from build123d import *

# Parameters (mm, degrees)
SKETCH1_R               = 60.625
SKETCH1_R_2             = 45
BOSS_EXTRUDE1_DEPTH     = 4
SKETCH2_R               = 49
SKETCH2_R_2             = 45
BOSS_EXTRUDE2_DEPTH     = 52
SKETCH4_W               = 13.25
SKETCH4_H               = 8
SKETCH4_W_2             = 8
SKETCH4_H_2             = 38
BOSS_EXTRUDE4_DEPTH     = 13
BOSS_EXTRUDE5_DEPTH     = 4
SKETCH7_R               = 1.3
CUT_EXTRUDE4_DEPTH      = 7.2
SKETCH9_W               = 10
SKETCH9_H               = 24
CUT_EXTRUDE7_DEPTH      = 8
CUT_EXTRUDE8_REACH      = 139.219
CUT_EXTRUDE8_END_RADIUS = 45
SKETCH11_R              = 5
CUT_EXTRUDE9_DEPTH      = 101.273532203


with BuildPart() as part:
    # Sketch1 → Boss-Extrude1 (new body)
    with BuildSketch(Plane(origin=(0, 0, 0), x_dir=(1, 0, 0), z_dir=(0, 1, 0))):
        with Locations(Location((0, 0, 0), (0, 0, 270))):
            Circle(SKETCH1_R)
        with Locations(Location((0, 0, 0), (0, 0, 270))):
            Circle(SKETCH1_R_2, mode=Mode.SUBTRACT)
    extrude(amount=BOSS_EXTRUDE1_DEPTH)

    # Sketch2 → Boss-Extrude2 (add)
    with BuildSketch(Plane(origin=(0, 4, 0), x_dir=(1, 0, 0), z_dir=(0, 1, 0))):
        with Locations(Location((0, 0, 0), (0, 0, 90))):
            Circle(SKETCH2_R)
        with Locations(Location((0, 0, 0), (0, 0, 270))):
            Circle(SKETCH2_R_2, mode=Mode.SUBTRACT)
    extrude(amount=BOSS_EXTRUDE2_DEPTH)

    # Sketch4 → Boss-Extrude4 (add, symmetric)
    with BuildSketch(Plane.XY):
        with Locations((-38.375, 34)):
            Rectangle(SKETCH4_W, SKETCH4_H)
        Polygon((-31.75, 30), (-45, 30), (-45, 16.75), align=None)
        with Locations((15.25, 19)):
            Rectangle(SKETCH4_W_2, SKETCH4_H_2)
    extrude(amount=BOSS_EXTRUDE4_DEPTH, both=True)


with BuildPart() as boss_extrude4_piece_1:
    # of the separate pieces the step leaves, piece 1, a body of its own (boss_extrude4_pieces)
    add(part.part.solids().sort_by_distance((0, 0, 60.625))[0])



with BuildPart() as boss_extrude4_piece_2:
    # of the separate pieces the step leaves, piece 2, a body of its own (boss_extrude4_pieces)
    add(part.part.solids().sort_by_distance((11.25, 38, -13))[0])


with BuildPart() as boss_extrude4_piece_1_1:
    add(boss_extrude4_piece_1.part)

    add(boss_extrude4_piece_2.part)  # Boss-Extrude5 merges Boss-Extrude4 piece 2
    # Sketch5 → Boss-Extrude5 (add)
    with BuildSketch(Plane.XZ):
        with BuildLine():
            Line((11.25, 13), (29.067400866, 34.352382842))
            ThreePointArc((29.067400866, 34.352382842), (45, 0), (29.067400866, -34.352382842))
            Line((29.067400866, -34.352382842), (11.25, -13))
            Line((11.25, -13), (11.25, 13))
        make_face()
    extrude(amount=-BOSS_EXTRUDE5_DEPTH)

    # Sketch7 → Cut-Extrude4 (cut)
    with BuildSketch(Plane(origin=(0, 38, 0), x_dir=(1, 0, 0), z_dir=(0, 1, 0))):
        with Locations(Location((-34.25, 5, 0), (0, 0, 180))):
            Circle(SKETCH7_R)
        with Locations(Location((-34.25, -5, 0), (0, 0, 180))):
            Circle(SKETCH7_R)
        with Locations(Location((13.75, 5, 0), (0, 0, 180))):
            Circle(SKETCH7_R)
        with Locations(Location((13.75, -5, 0), (0, 0, 180))):
            Circle(SKETCH7_R)
    extrude(amount=-CUT_EXTRUDE4_DEPTH, mode=Mode.SUBTRACT)

    # Sketch9 → Cut-Extrude7 (cut)
    with BuildSketch(Plane.ZY.offset(-11.25)):
        with Locations((0, 17)):
            Rectangle(SKETCH9_W, SKETCH9_H)
    extrude(amount=-CUT_EXTRUDE7_DEPTH, mode=Mode.SUBTRACT)

    # Cut-Extrude8: up to this cylinder (the profile starts outside it)
    cut_extrude8_end = Plane(origin=(0, 14, 0), z_dir=(0, -1, 0)) * Cylinder(CUT_EXTRUDE8_END_RADIUS, 369.438, mode=Mode.PRIVATE)
    # Sketch11 → Cut-Extrude8 (cut, up to the surface)
    with BuildSketch(Plane(origin=(49, 0, 0), x_dir=(0, 0, -1), z_dir=(1, 0, 0)), mode=Mode.PRIVATE) as cut_extrude8_sk1:
        with Locations((0, 14)):
            Circle(SKETCH11_R)
    cut_extrude8_tool1 = extrude(cut_extrude8_sk1.sketch, amount=-CUT_EXTRUDE8_REACH, mode=Mode.PRIVATE) - cut_extrude8_end
    add(cut_extrude8_tool1.solids().sort_by_distance((49, 14, 0))[0], mode=Mode.SUBTRACT)

    # Sketch12 → Cut-Extrude9 (cut, through all)
    with BuildSketch(Plane(origin=(0, 4, 0), x_dir=(1, 0, 0), z_dir=(0, 1, 0))):
        with BuildLine():
            Line((29.479537487, 22.359715328), (27.25, 19.687836398))
            Line((27.25, 19.687836398), (27.25, -19.687836398))
            Line((27.25, -19.687836398), (29.479537487, -22.359715328))
            ThreePointArc((29.479537487, -22.359715328), (37, 0), (29.479537487, 22.359715328))
        make_face()
        Polygon((27.25, -19.687836398), (27.25, 19.687836398), (24.25, 16.092634774), (24.25, -16.092634774), align=None)
    extrude(amount=-CUT_EXTRUDE9_DEPTH, mode=Mode.SUBTRACT)


solid = boss_extrude4_piece_1_1.part
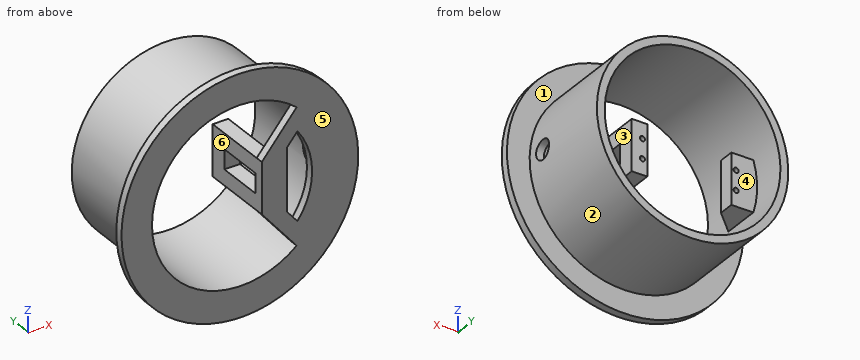
Design review of the part built by this model. Coordinates are the model's own, in mm. Face numbers are marked on the shaded views. A direction names the side the tool comes from. Give positions to 0.01 mm unless a question says otherwise; leave off trailing zeros. Loops run counter-clockwise (first coordinate to the right, second up) from the corner with the lowest first, then second, coordinate; pieces in that order, holes last. Notation, with made-up numbers: M 46.5,5 L 84.5,5 A35 cw 84.5,44 Z; hole C 23,-36.5 d11. An arc over 180 degrees is marked long. One line per question, with ' | ' between items. Start each with the question number.
1. To check wall thickness, follow L1, parallel to Z at x = -34.25, y = 36.25; L2, parallel to Y at x = -35.5, z = -43.5; L3, parallel to Z at x = 13, y = 32. State the ranges of each line that lie inside material, in increasing order.
2. The part is to be moulded in two halves that separate along X. For the marked faces 1, 2 and 3, say which applies: released by +X, released by -X, zero draft, split by the parting line, or undercut.
3. Insertion check: P1, Ø2, axis at x = 14, z = -5, coming from the +Y side; P2, Ø6, axis at x = -26.5, z = 4.5, coming from the -Y side; P3, Ø6, axis at x = -12, y = 50, coming from the +Z side; P4, Ø2, axis at x = -34.5, z = 5.5, coming from the +Y side. Each pin has a flat end and moves straight along its axis. Give the tip position at first contact, or say it passes through.
4. For the marked faces 4, 5 and 6, list the 3-axis set-ups (+Z, -Z, +X, -X, +Y, -Y) from which the entire face can be reached by the end or side of a thin tool; tool diameter is ignored.
5. Add section A-A (y = 24). Write out the cut boundary in (x, z), plus the area to 3 significant figures.
6. Add section C-C (z = 0). Give the number of separate pieces and of enclosed holes in the cut face, plus the area to 3 significant figures.
7. Add section B-B (x = 0). Write out the cut boundary in (y, z) (3 decimals), plus the area to 3 significant figures.
8. Add section D-D (z = -41.5). Write out the cut boundary in (x, y), plus the area to 3 significant figures.
Worked out:
1) L1: z = -35.04 to -29.19, -13 to -6.3, -3.7 to 3.7, 6.3 to 13, 29.19 to 35.04 | L2: y = 0 to 4 | L3: z = -47.24 to -43.08, -13 to -6.06, -3.94 to 3.94, 6.06 to 13, 43.08 to 47.24
2) face 1: zero draft | face 2: split by the parting line | face 3: undercut
3) P1: stops at y = 30.8 | P2: passes through | P3: stops at z = 48.17 | P4: stops at y = 38
4) face 4: +Y | face 5: +Z, -Z, +X, -X, -Y | face 6: +Y, -Y
5) outline: C 0,0 d98; M 11.25,-13 L 19.25,-13 L 19.25,-5 L 11.25,-5 Z; M 11.25,5 L 19.25,5 L 19.25,13 L 11.25,13 Z; hole M -43.08,-13 A45 ccw long -43.08,13 L -37.75,13 L -37.75,-13 Z | area: 1,480 mm²
6) separate pieces: 5 | enclosed holes: 0 | area: 859 mm²
7) outline: M 0,-60.625 L 4,-60.625 L 4,-49 L 56,-49 L 56,-45 L 0,-45 Z; M 0,45 L 56,45 L 56,49 L 4,49 L 4,60.625 L 0,60.625 Z | area: 541 mm²
8) outline: M -44.19,0 L -17.4,0 L -17.4,56 L -26.05,56 L -26.05,4 L -44.19,4 Z; M 17.4,0 L 44.19,0 L 44.19,4 L 26.05,4 L 26.05,56 L 17.4,56 Z | area: 1,110 mm²
